Check sheet for the modelled part. Datum: model origin and axes. Units: mm. Face numbers are marked on the shaded views. A direction names the side the tool comes from. Round coordinates to 2 decimals unless told otherwise and drop trailing zeros. Loops run counter-clockwise (first coordinate to the right, second up) from the corner with the lowest first, then second, coordinate; pieces in that order, holes last. Notation, with made-up numbers: (-21.5, 47.25) - (18.5, 47.25) arc R20 cw to (18.5, 75.25) - close; hole circle Ø5 at (-39, 47.5). An arc over 180 degrees is marked (long way). Put each result on its own line as item: value. Start each with the question number.
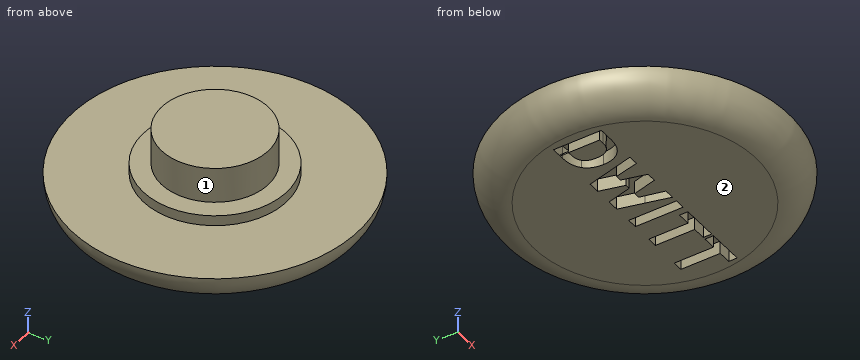
```python
from build123d import *

# Parameters (mm, degrees)
F0_R      = 11
F0_R_2    = 5.5
F1_DEPTH  = 2.5
F0_R_3    = 4.1
F2_DEPTH  = 3.3
F3_DEPTH  = 6.05
F4_R      = 2.49999
F7_W      = 0.7752131331
F7_H      = 1.8432312268
F7_H_2    = 1.8120306982
F8_DEPTH  = 1
F9_W      = 0.005
F9_H      = 0.6400108426
F10_DEPTH = 0.1


# Not quite as in the source:
# - a fillet or chamfer is up to 0.001 mm smaller than in the source, because OpenCascade refuses the exact size


with BuildPart() as f1:
    # F0 (on Top) → F1 (new body)
    with BuildSketch(Plane.XY):
        Circle(F0_R)
        Circle(F0_R_2, mode=Mode.SUBTRACT)
    extrude(amount=F1_DEPTH)

    # F0 (on Top) → F2 (join, through all)
    with BuildSketch(Plane.XY):
        Circle(F0_R_2)
        Circle(F0_R_3, mode=Mode.SUBTRACT)
    extrude(amount=F2_DEPTH)

    # F0 (on Top) → F3 (join, through all)
    with BuildSketch(Plane.XY):
        Circle(F0_R_3)
    extrude(amount=F3_DEPTH)

    # F4 (radius 2.5 in the source; OpenCascade refuses exactly that, so slightly less here)
    f4_edges = [f1.edges().sort_by_distance(p)[0] for p in [
        (-11, 0, 0),
    ]]
    fillet(f4_edges, radius=F4_R)

    # F7 (on face) → F8 (cut)
    with BuildSketch(Plane(origin=(0, 0, 0), x_dir=(1, 0, 0), z_dir=(0, 0, -1))):
        with BuildLine():
            Line((-7.8377327815, 1.8120306982), (-7.8377327815, 0))
            Line((-7.8377327815, 0), (-7.0625196484, 0))
            Line((-7.0625196484, 0), (-7.0625196484, 1.1768199369))
            Line((-7.0625196484, 1.1768199369), (-6.6505126685, 1.1768199369))
            add(Edge.make_bspline(
                [(-5.6104951692, 0), (-5.6108483761, 1.1768199369), (-6.6505126685, 1.1768199369)],
                knots=[0.0003397316, 0.0003397316, 0.0003397316, 1, 1, 1], degree=2))
            Line((-5.6104951692, 0), (-4.8049398646, 0))
            add(Edge.make_bspline(
                [(-4.804881401, 0.0192003253), (-4.804881401, 0.0095761402), (-4.8049398646, 0)],
                knots=[0, 0, 0, 0.010664918, 0.010664918, 0.010664918], degree=2))
            add(Edge.make_bspline(
                [(-5.3000897905, 1.339622695), (-4.804881401, 0.8672146918), (-4.804881401, 0.0192003253)],
                knots=[0, 0, 0, 1, 1, 1], degree=2))
            add(Edge.make_bspline(
                [(-6.6905133461, 1.8120306982), (-5.79529818, 1.8120306982), (-5.3000897905, 1.339622695)],
                knots=[0, 0, 0, 1, 1, 1], degree=2))
            Line((-6.6905133461, 1.8120306982), (-7.8377327815, 1.8120306982))
        make_face()
        with BuildLine():
            Line((-7.0625196484, 0), (-7.8377327815, 0))
            Line((-7.8377327815, 0), (-7.8377327815, -1.8432312268))
            Line((-7.8377327815, -1.8432312268), (-6.8025152436, -1.8432312268))
            add(Edge.make_bspline(
                [(-5.318890109, -1.3632230948), (-5.832898817, -1.8432312268), (-6.8025152436, -1.8432312268)],
                knots=[0, 0, 0, 1, 1, 1], degree=2))
            add(Edge.make_bspline(
                [(-4.8049398646, 0), (-4.8103632617, -0.8883342102), (-5.318890109, -1.3632230948)],
                knots=[0.010664918, 0.010664918, 0.010664918, 1, 1, 1], degree=2))
            Line((-4.8049398646, 0), (-5.6104951692, 0))
            add(Edge.make_bspline(
                [(-5.6104950492, -0.0008000136), (-5.6104950492, -0.0003999388), (-5.6104951692, 0)],
                knots=[0, 0, 0, 0.0003397316, 0.0003397316, 0.0003397316], degree=2))
            add(Edge.make_bspline(
                [(-6.7305140238, -1.2032203841), (-5.6104950492, -1.2032203841), (-5.6104950492, -0.0008000136)],
                knots=[0, 0, 0, 1, 1, 1], degree=2))
            Line((-6.7305140238, -1.2032203841), (-7.0625196484, -1.2032203841))
            Line((-7.0625196484, -1.2032203841), (-7.0625196484, 0))
        make_face()
        Polygon((6.1985050109, 1.1672197742), (6.1985050109, 0), (6.973718144, 0), (6.973718144, 1.1672197742), (7.9657349501, 1.1672197742), (7.9657349501, 1.8120306982), (5.2056881912, 1.8120306982), (5.2056881912, 1.1672197742), align=None)
        with Locations((6.5861115774, -0.9216156134)):
            Rectangle(F7_W, F7_H)
        Polygon((3.2336547824, 1.1672197742), (3.2336547824, 0), (4.0088679155, 0), (4.0088679155, 1.1672197742), (5.0008847216, 1.1672197742), (5.0008847216, 1.8120306982), (2.2408379628, 1.8120306982), (2.2408379628, 1.1672197742), align=None)
        with Locations((3.6212613489, -0.9216156134)):
            Rectangle(F7_W, F7_H)
        with Locations((1.2908218682, 0.9060153491)):
            Rectangle(F7_W, F7_H_2)
        with Locations((1.2908218682, -0.9216156134)):
            Rectangle(F7_W, F7_H)
        Polygon((-4.5072763592, 1.8120306982), (-4.044849615, 0), (-3.3198281749, 0), (-3.7448634429, 1.8120306982), align=None)
        with BuildLine():
            Line((-3.3198281749, 0), (-4.044849615, 0))
            Line((-4.044849615, 0), (-3.5744605561, -1.8432312268))
            Line((-3.5744605561, -1.8432312268), (-2.6944456475, -1.8432312268))
            Line((-2.6944456475, -1.8432312268), (-2.2209338662, 0))
            Line((-2.2209338662, 0), (-2.868251717, 0))
            Line((-2.868251717, 0), (-2.9296496321, -0.2360039982))
            add(Edge.make_bspline(
                [(-3.0308513466, -0.6996118523), (-2.9768504318, -0.4008067902), (-2.9296496321, -0.2360039982)],
                knots=[0, 0, 0, 1, 1, 1], degree=2))
            add(Edge.make_bspline(
                [(-3.100052519, -1.140819327), (-3.0848522615, -0.9984169145), (-3.0308513466, -0.6996118523)],
                knots=[0, 0, 0, 1, 1, 1], degree=2))
            add(Edge.make_bspline(
                [(-3.2768555143, -0.1832031037), (-3.1544534406, -0.736012469), (-3.100052519, -1.140819327)],
                knots=[0, 0, 0, 1, 1, 1], degree=2))
            Line((-3.2768555143, -0.1832031037), (-3.3198281749, 0))
        make_face()
        with BuildLine():
            Line((-2.868251717, 0), (-3.3198281749, 0))
            Line((-3.3198281749, 0), (-3.2768555143, -0.1832031037))
            add(Edge.make_bspline(
                [(-3.2768555143, -0.1832031037), (-3.1544534406, -0.736012469), (-3.100052519, -1.140819327)],
                knots=[0, 0, 0, 1, 1, 1], degree=2))
            add(Edge.make_bspline(
                [(-3.100052519, -1.140819327), (-3.0848522615, -0.9984169145), (-3.0308513466, -0.6996118523)],
                knots=[0, 0, 0, 1, 1, 1], degree=2))
            add(Edge.make_bspline(
                [(-3.0308513466, -0.6996118523), (-2.9768504318, -0.4008067902), (-2.9296496321, -0.2360039982)],
                knots=[0, 0, 0, 1, 1, 1], degree=2))
            Line((-2.9296496321, -0.2360039982), (-2.868251717, 0))
        make_face()
        with BuildLine():
            Line((-2.3968406056, 1.8120306982), (-2.868251717, 0))
            Line((-2.868251717, 0), (-2.2209338662, 0))
            Line((-2.2209338662, 0), (-2.2024373122, 0.0720012198))
            add(Edge.make_bspline(
                [(-2.10963574, 0.4980084369), (-2.1696367565, 0.1992033748), (-2.2024373122, 0.0720012198)],
                knots=[0, 0, 0, 1, 1, 1], degree=2))
            add(Edge.make_bspline(
                [(-2.034434466, 0.9320157896), (-2.0496347235, 0.7968134991), (-2.10963574, 0.4980084369)],
                knots=[0, 0, 0, 1, 1, 1], degree=2))
            add(Edge.make_bspline(
                [(-1.9584331784, 0.5004084776), (-2.0248343034, 0.8216139192), (-2.034434466, 0.9320157896)],
                knots=[0, 0, 0, 1, 1, 1], degree=2))
            add(Edge.make_bspline(
                [(-1.8648315927, 0.0768013011), (-1.8920320535, 0.1792030359), (-1.9584331784, 0.5004084776)],
                knots=[0, 0, 0, 1, 1, 1], degree=2))
            Line((-1.8648315927, 0.0768013011), (-1.8450232571, 0))
            Line((-1.8450232571, 0), (-1.1934170931, 0))
            Line((-1.1934170931, 0), (-1.6648282044, 1.8120306982))
            Line((-1.6648282044, 1.8120306982), (-2.3968406056, 1.8120306982))
        make_face()
        with BuildLine():
            Line((-2.2024373122, 0.0720012198), (-2.2209338662, 0))
            Line((-2.2209338662, 0), (-1.8450232571, 0))
            Line((-1.8450232571, 0), (-1.8648315927, 0.0768013011))
            add(Edge.make_bspline(
                [(-1.8648315927, 0.0768013011), (-1.8920320535, 0.1792030359), (-1.9584331784, 0.5004084776)],
                knots=[0, 0, 0, 1, 1, 1], degree=2))
            add(Edge.make_bspline(
                [(-1.9584331784, 0.5004084776), (-2.0248343034, 0.8216139192), (-2.034434466, 0.9320157896)],
                knots=[0, 0, 0, 1, 1, 1], degree=2))
            add(Edge.make_bspline(
                [(-2.034434466, 0.9320157896), (-2.0496347235, 0.7968134991), (-2.10963574, 0.4980084369)],
                knots=[0, 0, 0, 1, 1, 1], degree=2))
            add(Edge.make_bspline(
                [(-2.10963574, 0.4980084369), (-2.1696367565, 0.1992033748), (-2.2024373122, 0.0720012198)],
                knots=[0, 0, 0, 1, 1, 1], degree=2))
        make_face()
        with BuildLine():
            Line((-1.1934170931, 0), (-1.8450232571, 0))
            Line((-1.8450232571, 0), (-1.3696232032, -1.8432312268))
            Line((-1.3696232032, -1.8432312268), (-0.487208254, -1.8432312268))
            Line((-0.487208254, -1.8432312268), (-0.0180294584, 0))
            Line((-0.0180294584, 0), (-0.7421344653, 0))
            Line((-0.7421344653, 0), (-0.7848132958, -0.1832031037))
            add(Edge.make_bspline(
                [(-0.8848149899, -0.6544110866), (-0.8296140548, -0.3632061532), (-0.7848132958, -0.1832031037)],
                knots=[0, 0, 0, 1, 1, 1], degree=2))
            add(Edge.make_bspline(
                [(-0.9648163453, -1.140819327), (-0.9400159251, -0.94561602), (-0.8848149899, -0.6544110866)],
                knots=[0, 0, 0, 1, 1, 1], degree=2))
            add(Edge.make_bspline(
                [(-1.0444176938, -0.6556111069), (-0.9920168061, -0.938415898), (-0.9648163453, -1.140819327)],
                knots=[0, 0, 0, 1, 1, 1], degree=2))
            add(Edge.make_bspline(
                [(-1.1320191779, -0.2360039982), (-1.0968185816, -0.3728063158), (-1.0444176938, -0.6556111069)],
                knots=[0, 0, 0, 1, 1, 1], degree=2))
            Line((-1.1320191779, -0.2360039982), (-1.1934170931, 0))
        make_face()
        with BuildLine():
            Line((-0.7421344653, 0), (-1.1934170931, 0))
            Line((-1.1934170931, 0), (-1.1320191779, -0.2360039982))
            add(Edge.make_bspline(
                [(-1.1320191779, -0.2360039982), (-1.0968185816, -0.3728063158), (-1.0444176938, -0.6556111069)],
                knots=[0, 0, 0, 1, 1, 1], degree=2))
            add(Edge.make_bspline(
                [(-1.0444176938, -0.6556111069), (-0.9920168061, -0.938415898), (-0.9648163453, -1.140819327)],
                knots=[0, 0, 0, 1, 1, 1], degree=2))
            add(Edge.make_bspline(
                [(-0.9648163453, -1.140819327), (-0.9400159251, -0.94561602), (-0.8848149899, -0.6544110866)],
                knots=[0, 0, 0, 1, 1, 1], degree=2))
            add(Edge.make_bspline(
                [(-0.8848149899, -0.6544110866), (-0.8296140548, -0.3632061532), (-0.7848132958, -0.1832031037)],
                knots=[0, 0, 0, 1, 1, 1], degree=2))
            Line((-0.7848132958, -0.1832031037), (-0.7421344653, 0))
        make_face()
        Polygon((-0.3200054213, 1.8120306982), (-0.7421344653, 0), (-0.0180294584, 0), (0.4432075085, 1.8120306982), align=None)
    extrude(amount=-F8_DEPTH, mode=Mode.SUBTRACT)

    # F9 (on face) → F10 (join)
    with BuildSketch(Plane(origin=(0, 0, 0), x_dir=(1, 0, 0), z_dir=(0, 0, -1))):
        with Locations((-7.0600196484, -1.5232258055)):
            Rectangle(F9_W, F9_H)
    extrude(amount=-F10_DEPTH)


solid = f1.part
```
Q1. Cross-section at C-C on z = 2. Enter the section's corners in (x, y).
Q2. Cross-section at A-A on z = 0.5. State how many separate pieces and enclosed holes the cut face has, and give its area (3 significant figures).
Q3. Material ranges on line 1 (Y direction, x = -5.75, z = 0.5); line 2 (Z direction, x = 5, y = 3.25); line 3 (X direction, y = -6.75, z = 0.75), recorded low to high. Write a range as from..to.
Q4. Set-up check for the marked faces 1 and 2: record each of +Z, -Z, +X, -X, +Y, -Y from which the full face is reachable in a straight line by a thin tool's end or side.
Q5. Depth check by flat-ended pin: pin 1 Ø0.5 at (y, z) = (0.5, 0.5) entering from -X; pin 2 Ø3 at (x, z) = (1.5, 5) entering from -Y; pin 3 Ø0.8 at (x, z) = (4, 0.5) entering from +Y. Enter the tip coordinate at first touch or a pass-through.
Q6. Cross-section at B-B on z = 4.75. Enter the section's corners in (x, y), and give its area (3 significant figures).
Answer list:
1. outline: circle Ø21.9 at (0, 0)
2. separate pieces: 2
2. enclosed holes: 5
2. area: 286 mm2
3. line 1: y = -8.18..-1.64, -0.7..0.7, 1.65..8.18
3. line 2: z = 0..2.5
3. line 3: x = -7.76..7.76
4. face 1: +Z
4. face 2: -Z, +X, -X, +Y, -Y
5. pin 1: stops at x = -10.27
5. pin 2: stops at y = -4.1
5. pin 3: stops at y = 9.66
6. outline: circle Ø8.2 at (0, 0)
6. area: 52.8 mm2
